```python
from build123d import *

# Parameters (mm, degrees)
SKETCH1_W                                           = 107
SKETCH1_H                                           = 26
BOSS_EXTRUDE1_DEPTH                                 = 15
SKETCH2_W                                           = 1
SKETCH2_H                                           = 14.5
SKETCH2_W_2                                         = 6
SKETCH2_H_2                                         = 13.5
CUT_EXTRUDE1_DEPTH                                  = 112.130553854
FILLET1_R                                           = 0.5
CSK_FOR_M2_COUNTERSUNK_FLAT_HEAD_SCREW1_D           = 2.4
CSK_FOR_M2_COUNTERSUNK_FLAT_HEAD_SCREW1_DEPTH       = 15
CSK_FOR_M2_COUNTERSUNK_FLAT_HEAD_SCREW1_CSINK_D     = 4.4
CSK_FOR_M2_COUNTERSUNK_FLAT_HEAD_SCREW1_CSINK_ANGLE = 90
CSK_FOR_M2_COUNTERSUNK_FLAT_HEAD_SCREW1_TIP         = 0.721032743
SKETCH14_W                                          = 97
SKETCH14_H                                          = 24
CUT_EXTRUDE7_DEPTH                                  = 112.130553854
SKETCH14_3_W                                        = 97
SKETCH14_3_H                                        = 24
BOSS_EXTRUDE3_DEPTH                                 = 1
SKETCH18_W                                          = 97
SKETCH18_H                                          = 24
CUT_EXTRUDE8_DEPTH                                  = 112.130553854
SKETCH20_W                                          = 97
SKETCH20_H                                          = 24
SKETCH20_W_2                                        = 93
SKETCH20_H_2                                        = 20
BOSS_EXTRUDE4_DEPTH                                 = 15
SKETCH20_2_W                                        = 97
SKETCH20_2_H                                        = 24
SKETCH20_2_W_2                                      = 93
SKETCH20_2_H_2                                      = 20
CUT_EXTRUDE9_DEPTH                                  = 3
SKETCH21_W                                          = 52
SKETCH21_H                                          = 2
BOSS_EXTRUDE5_DEPTH                                 = 5
SKETCH22_W                                          = 52
SKETCH22_H                                          = 2
BOSS_EXTRUDE6_DEPTH                                 = 5
SKETCH23_W                                          = 0.5
SKETCH23_H                                          = 16.612240618
CUT_EXTRUDE10_DEPTH                                 = 112.130553854
BOSS_EXTRUDE7_REACH                                 = 111.983
SKETCH25_W                                          = 2
SKETCH25_H                                          = 12
CUT_EXTRUDE11_REACH                                 = 65.537
SKETCH26_W                                          = 10
SKETCH26_H                                          = 2


with BuildPart() as part:
    # Sketch1 → Boss-Extrude1 (new body)
    with BuildSketch(Plane(origin=(0, 0, 0), x_dir=(1, 0, 0), z_dir=(0, 1, 0))):
        with Locations((53.5, -13)):
            Rectangle(SKETCH1_W, SKETCH1_H)
    extrude(amount=BOSS_EXTRUDE1_DEPTH)

    # Sketch2 → Cut-Extrude1 (cut, through all)
    with BuildSketch(Plane.XY.offset(26)):
        with Locations((106.5, 7.75)):
            Rectangle(SKETCH2_W, SKETCH2_H)
        with Locations((3, 8.25)):
            Rectangle(SKETCH2_W_2, SKETCH2_H_2)
    extrude(amount=-CUT_EXTRUDE1_DEPTH, mode=Mode.SUBTRACT)

    # Fillet1
    fillet1_edges = [part.edges().sort_by_distance(p)[0] for p in [
        (106, 15, 13),
        (0, 1.5, 13),
        (6, 15, 13),
    ]]
    fillet(fillet1_edges, radius=FILLET1_R)

    # CSK for M2 Countersunk Flat Head Screw1
    with Locations(Plane(origin=(3, 1.5, 13), x_dir=(1, 0, 0), z_dir=(0, 1, 0))):
        with Locations((0, 0)):
            CounterSinkHole(CSK_FOR_M2_COUNTERSUNK_FLAT_HEAD_SCREW1_D / 2, CSK_FOR_M2_COUNTERSUNK_FLAT_HEAD_SCREW1_CSINK_D / 2, depth=CSK_FOR_M2_COUNTERSUNK_FLAT_HEAD_SCREW1_DEPTH, counter_sink_angle=CSK_FOR_M2_COUNTERSUNK_FLAT_HEAD_SCREW1_CSINK_ANGLE)
            with Locations((0, 0, -(CSK_FOR_M2_COUNTERSUNK_FLAT_HEAD_SCREW1_DEPTH + CSK_FOR_M2_COUNTERSUNK_FLAT_HEAD_SCREW1_TIP / 2))):  # 118° drill point
                Cone(0, CSK_FOR_M2_COUNTERSUNK_FLAT_HEAD_SCREW1_D / 2, CSK_FOR_M2_COUNTERSUNK_FLAT_HEAD_SCREW1_TIP, mode=Mode.SUBTRACT)

    # Sketch14 → Cut-Extrude7 (cut, through all)
    with BuildSketch(Plane(origin=(0, 15, 0), x_dir=(1, 0, 0), z_dir=(0, 1, 0))):
        with Locations((56, -13)):
            Rectangle(SKETCH14_W, SKETCH14_H)
    extrude(amount=-CUT_EXTRUDE7_DEPTH, mode=Mode.SUBTRACT)

    # Sketch14<3> → Boss-Extrude3 (add)
    with BuildSketch(Plane(origin=(0, 15, 0), x_dir=(1, 0, 0), z_dir=(0, 1, 0))):
        with Locations((56, -13)):
            Rectangle(SKETCH14_3_W, SKETCH14_3_H)
    extrude(amount=-BOSS_EXTRUDE3_DEPTH)

    # Sketch18 → Cut-Extrude8 (cut, through all)
    with BuildSketch(Plane(origin=(0, 0, 0), x_dir=(1, 0, 0), z_dir=(0, 1, 0))):
        with Locations((56, -13)):
            Rectangle(SKETCH18_W, SKETCH18_H)
    extrude(amount=CUT_EXTRUDE8_DEPTH, mode=Mode.SUBTRACT)

    # Sketch20 → Boss-Extrude4 (add)
    with BuildSketch(Plane(origin=(0, 15, 0), x_dir=(1, 0, 0), z_dir=(0, 1, 0))):
        with Locations((56, -13)):
            Rectangle(SKETCH20_W, SKETCH20_H)
        with Locations((56, -13)):
            Rectangle(SKETCH20_W_2, SKETCH20_H_2, mode=Mode.SUBTRACT)
    extrude(amount=-BOSS_EXTRUDE4_DEPTH)

    # Sketch20<2> → Cut-Extrude9 (cut)
    with BuildSketch(Plane(origin=(0, 15, 0), x_dir=(1, 0, 0), z_dir=(0, 1, 0))):
        with Locations((56, -13)):
            Rectangle(SKETCH20_2_W, SKETCH20_2_H)
        with Locations((56, -13)):
            Rectangle(SKETCH20_2_W_2, SKETCH20_2_H_2, mode=Mode.SUBTRACT)
    extrude(amount=-CUT_EXTRUDE9_DEPTH, mode=Mode.SUBTRACT)

    # Sketch21 → Boss-Extrude5 (add)
    with BuildSketch(Plane.XY.offset(3)):
        with Locations((76.5, 1)):
            Rectangle(SKETCH21_W, SKETCH21_H)
    extrude(amount=BOSS_EXTRUDE5_DEPTH)

    # Sketch22 → Boss-Extrude6 (add)
    with BuildSketch(Plane(origin=(0, 0, 23), x_dir=(-1, 0, 0), z_dir=(0, 0, -1))):
        with Locations((-76.5, 1)):
            Rectangle(SKETCH22_W, SKETCH22_H)
    extrude(amount=BOSS_EXTRUDE6_DEPTH)

    # Sketch23 → Cut-Extrude10 (cut, through all)
    with BuildSketch(Plane.XY.offset(26)):
        with Locations((106.75, 8.306120309)):
            Rectangle(SKETCH23_W, SKETCH23_H)
    extrude(amount=-CUT_EXTRUDE10_DEPTH, mode=Mode.SUBTRACT)

    # Sketch25 → Boss-Extrude7 (add, up to next)
    with BuildSketch(Plane(origin=(0, 0, 23), x_dir=(-1, 0, 0), z_dir=(0, 0, -1)), mode=Mode.PRIVATE) as boss_extrude7_sk1:
        with Locations((-49.5, 6)):
            Rectangle(SKETCH25_W, SKETCH25_H)
    boss_extrude7_tool1 = extrude(boss_extrude7_sk1.sketch, amount=BOSS_EXTRUDE7_REACH, mode=Mode.PRIVATE) - part.part
    add(boss_extrude7_tool1.solids().sort_by_distance((49.5, 6, 23))[0])

    # Sketch26 → Cut-Extrude11 (cut, up to next)
    with BuildSketch(Plane(origin=(50.5, 0, 0), x_dir=(0, 0, -1), z_dir=(1, 0, 0)), mode=Mode.PRIVATE) as cut_extrude11_sk1:
        with Locations((-13, 1)):
            Rectangle(SKETCH26_W, SKETCH26_H)
    cut_extrude11_tool1 = extrude(cut_extrude11_sk1.sketch, amount=-CUT_EXTRUDE11_REACH, mode=Mode.PRIVATE) & part.part
    add(cut_extrude11_tool1.solids().sort_by_distance((50.5, 1, 13))[0], mode=Mode.SUBTRACT)


solid = part.part
```
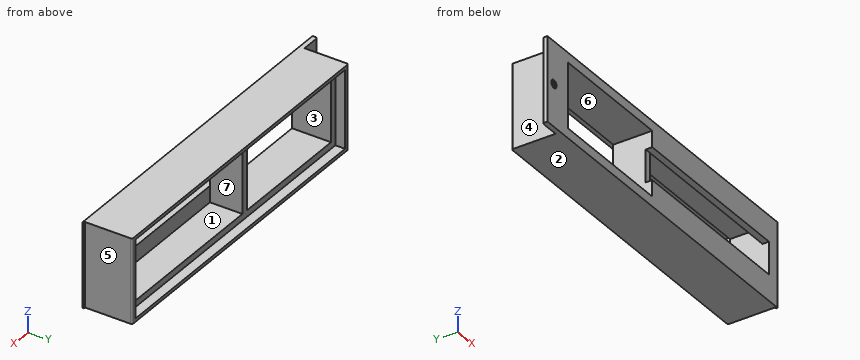
Source: CAD feature listing. Evaluate the final solid. Frame: model axes, mm. Face numbers are marked on the shaded views. A direction names the side the tool comes from. Round coordinates to 2 decimals unless told otherwise and drop trailing zeros. Loops run counter-clockwise (first coordinate to the right, second up) from the corner with the lowest first, then second, coordinate; pieces in that order, holes last. Notation, with made-up numbers: M 84.25,67.5 L 130.25,67.5 A38 cw 130.25,106.5 Z; hole C 63.5,80.5 d7. An arc over 180 degrees is marked long. Put each result on its own line as item: value.
(1) Access query for the marked faces 5, 6 and 7. Directions: +Z, -Z, +X, -X, +Y, -Y. A direction counts if a zero-diameter tool reaches every point of the face in a straight line with its end or side. Return the directions, or none.
Solutions:
face 5: +Z, -Z, +X, +Y
face 6: +Y, -Y
face 7: +Y
(2) Section A-A, the plane z = 13. State how many separate pieces and enclosed holes the cut face has, and give its area (3 significant figures).
Solutions:
separate pieces: 4
enclosed holes: 0
area: 117 mm²
(3) Ray query, line 1 (X direction, y = 0.1, z = 13); line 2 (X direction, y = 6.5, z = 11); line 3 (Z direction, x = 45, y = 3.5). Return the intervals inside material, ascending. Write a range as [from, to].
Solutions:
line 1: [0, 1.8], [4.2, 9.5], [102.5, 106.5]
line 2: [6, 9.5], [48.5, 50.5], [102.5, 106]
line 3: [0, 3], [23, 26]
(4) Pull-direction query (X, two-part tool) for the marked faces 1, 2, 3 and 4; classes: released by +X, released by -X, zero draft, split by the parting line, or undercut.
Solutions:
face 1: undercut
face 2: zero draft
face 3: undercut
face 4: released by -X
(5) Section B-B, the plane x = 12.5. Return loops of the section in (y, z), and give its area (3 significant figures).
Solutions:
outline: M 0,0 L 15,0 L 15,1 L 12,1 L 12,3 L 0,3 Z; M 0,23 L 12,23 L 12,25 L 15,25 L 15,26 L 0,26 Z
area: 78.0 mm²
(6) First-contact query: pin 1 (3 mm diameter, centred on x = 71, z = 3.5, fed in from -Y); pin 2 (4 mm diameter, centred on x = 79.5, z = 19.5, fed in from +Y); pin 3 (6.5 mm diameter, centred on y = 6.5, z = 12, fed in from -X); pin 4 (0.6 mm diameter, centred on x = 50, z = 13.5, fed in from -Y). Flat tips, straight axial feed; report the tip coordinate or a pass-through.
Solutions:
pin 1: y = 0
pin 2: y = 2
pin 3: x = 6
pin 4: y = 2
(7) Section C-C, the plane y = 5.25. Return loops of the section in (x, z).
Solutions:
outline: M 6,0 L 106,0 L 106,26 L 6,26 Z; hole M 9.5,3 L 48.5,3 L 48.5,23 L 9.5,23 Z; hole M 50.5,3 L 102.5,3 L 102.5,23 L 50.5,23 Z
